Source: three-view drawing plus pictorial views. Frame: mm from the lowest corner of the part. Coordinates: 2 decimals unless noted, no trailing zeros. Write each loop counter-clockwise with the first axis right and the second up, starting at its lowest first coordinate (ties: lowest second). Pieces come first, ordered by that corner, then holes. Notation, with made-up numbers: (-27.75, 9.25) - (27.25, 9.25) arc R26 ccw to (27.25, 38.25) - close; hole circle Ø5 at (89, -15). An arc over 180 degrees is marked (long way). Put each result on its own line as item: value. Start each with the question number.
1. Pin query (flat end, axial travel): pin 1 (3 mm diameter, centred on x = 22.5, z = 72, fed in from -Y); pin 2 (2.5 mm diameter, centred on y = 52.5, z = 70, fed in from +X); pin 3 (2 mm diameter, centred on y = 24, z = 19.5, fed in from -X). Return the tip coordinate at first contact, or that it passes through.
2. Cut plane B-B, the plane x = 57. Return loops of the section in (y, z) (1 decimal), and give its area (3 significant figures).
3. Line query: line 1 (Y direction, x = 105.5, z = 67); line 2 (Y direction, x = 19, z = 73); line 3 (Z direction, x = 72, y = 53.5) (1 decimal). Output: solid intervals per line, ascending.
4. Cut plane D-D, the plane y = 45.5. Return loops of the section in (x, z) (1 decimal).
5. Cut plane A-A, the plane z = 70.5. Return loops of the section in (x, y) (1 decimal), and give its area (3 significant figures).
6. Cut plane C-C, the plane x = 31. Return loops of the section in (y, z) (1 decimal), and give its area (3 significant figures).
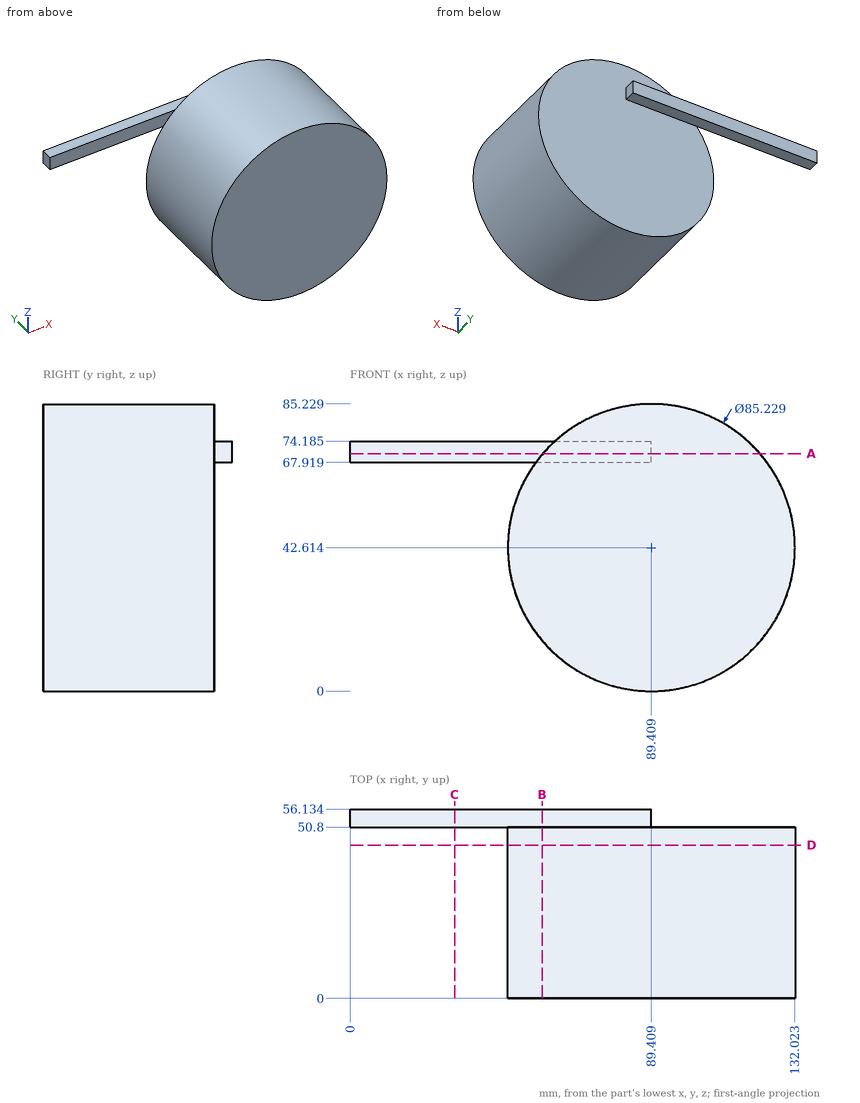
Report:
1. pin 1: stops at y = 50.8
1. pin 2: stops at x = 89.41
1. pin 3: stops at x = 52.98
2. outline: (0, 14.9) - (50.8, 14.9) - (50.8, 67.9) - (56.1, 67.9) - (56.1, 74.2) - (50.8, 74.2) - (50.8, 70.3) - (0, 70.3) - close
2. area: 2,840 mm^2
3. line 1: y = 0 to 50.8
3. line 2: y = 50.8 to 56.13
3. line 3: z = 67.9 to 74.2
4. outline: circle Ø85.2 at (89.4, 42.6)
5. outline: (0, 50.8) - (57.2, 50.8) - (57.2, 0) - (121.6, 0) - (121.6, 50.8) - (89.4, 50.8) - (89.4, 56.1) - (0, 56.1) - close
5. area: 3,750 mm^2
6. outline: (50.8, 67.9) - (56.1, 67.9) - (56.1, 74.2) - (50.8, 74.2) - close
6. area: 33.4 mm^2
